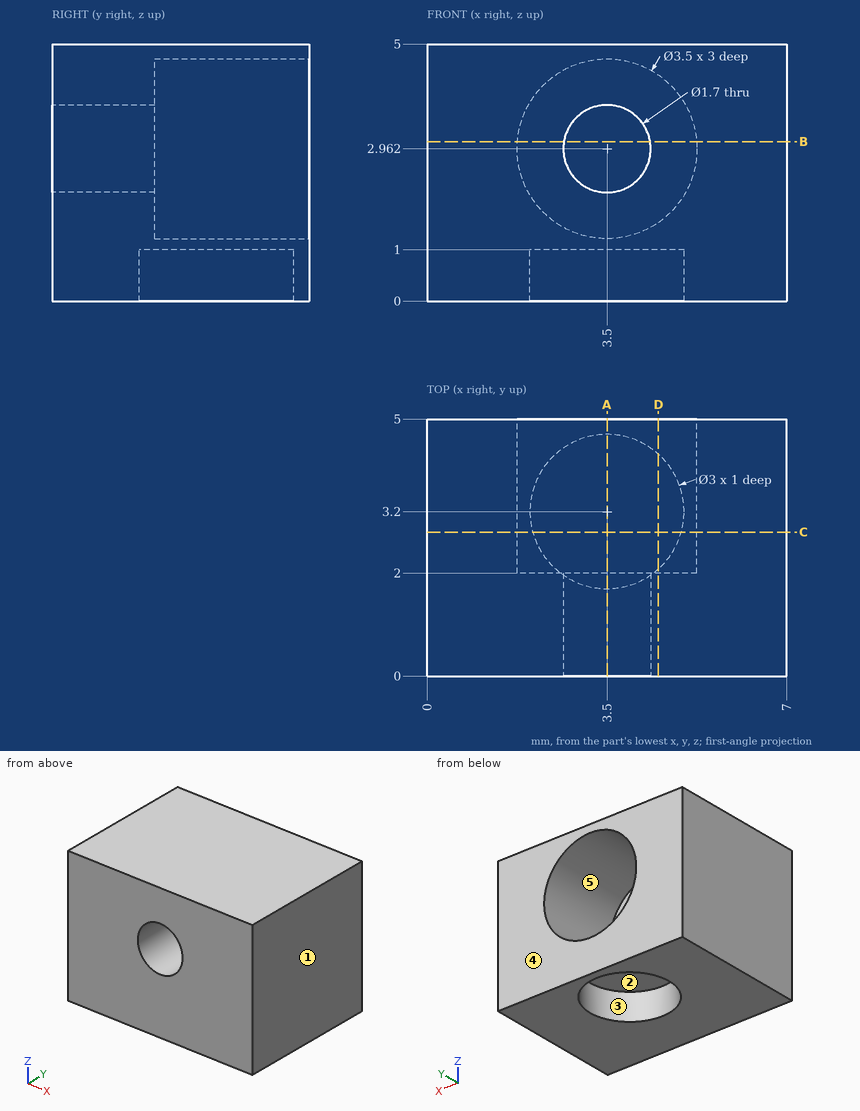
Can you work these out from the drawing? Everything is in mm from the part's minimum corner. A direction names the side the tool comes from. Coordinates: 2 decimals unless noted, no trailing zeros. Loops run counter-clockwise (first coordinate to the right, second up) from the corner with the lowest first, then second, coordinate; pieces in that order, holes last.
1) For pin 1 (1.7 mm diameter, centred on x = 4, z = 2.5, fed in from +Y); pin 2 (1.5 mm diameter, centred on x = 3, y = 3, fed in from -Z); pin 3 (1.5 mm diameter, centred on x = 3.5, z = 2.96, fed in from +Y), each with a flat end and sliding along its axis, tell me the tip position at first contact or that it passes through.
2) Imagine slicing it at A-A on x = 3.5. List the corners of the cut face in (y, z) for me, plus the area to 3 significant figures.
3) Imagine slicing it at B-B on z = 3.1. List the corners of the cut face in (x, y) for me.
4) Which directions (+Z, -Z, +X, -X, +Y, -Y) give clear straight access to the entire face, cutting with the end or side of a thin tool? Please do the marked faces 1 and 2.
5) Thinking about a two-plate mould opening in Y: for the marked faces 3, 4 and 5, which applies, pulls with the +Y half, pulls with the -Y half, needs draft (parallel to the pull), parting line crosses it, or undercut?
6) I need wall thicknesses on probe 1 along X at (y, z) = (1.7, 2.9); probe 2 along Z at (x, y) = (3.5, 2.75); probe 3 along Y at (x, z) = (3.5, 0.55). Which ranges of each line are inside material? Lowest first, please.
7) Imagine slicing it at D-D on x = 4.5. List the corners of the cut face in (y, z) for me.
8) Imagine slicing it at C-C on y = 2.8. List the corners of the cut face in (x, z) for me.
Completed:
1. pin 1: stops at y = 2
1. pin 2: stops at z = 1
1. pin 3: passes through
2. outline: (0, 0) - (1.7, 0) - (1.7, 1) - (4.7, 1) - (4.7, 0) - (5, 0) - (5, 1.21) - (2, 1.21) - (2, 2.11) - (0, 2.11) - close; (0, 3.81) - (2, 3.81) - (2, 4.71) - (5, 4.71) - (5, 5) - (0, 5) - close
2. area: 8.10 mm2
3. outline: (0, 0) - (2.66, 0) - (2.66, 2) - (1.76, 2) - (1.76, 5) - (0, 5) - close; (4.34, 0) - (7, 0) - (7, 5) - (5.24, 5) - (5.24, 2) - (4.34, 2) - close
4. face 1: +Z, -Z, +X, +Y, -Y
4. face 2: -Z
5. face 3: undercut
5. face 4: pulls with the +Y half
5. face 5: needs draft
6. probe 1: x = 0 to 2.65, 4.35 to 7
6. probe 2: z = 1 to 1.21, 4.71 to 5
6. probe 3: y = 0 to 1.7, 4.7 to 5
7. outline: (0, 0) - (2.08, 0) - (2.08, 1) - (4.32, 1) - (4.32, 0) - (5, 0) - (5, 1.53) - (2, 1.53) - (2, 4.4) - (5, 4.4) - (5, 5) - (0, 5) - close
8. outline: (0, 0) - (2.05, 0) - (2.05, 1) - (4.95, 1) - (4.95, 0) - (7, 0) - (7, 5) - (0, 5) - close; hole circle Ø3.5 at (3.5, 2.96)
